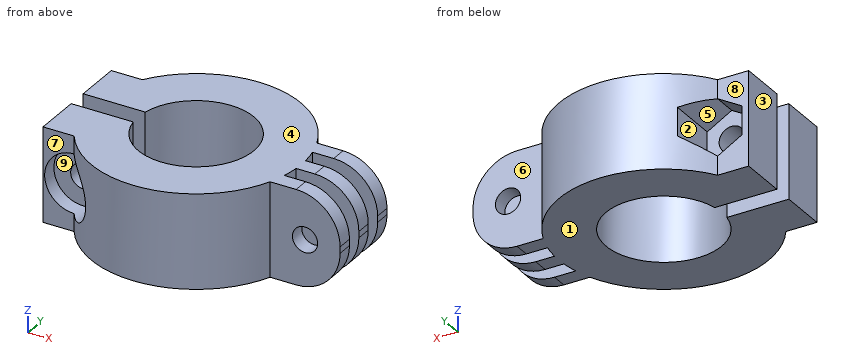
```python
from build123d import *

# Parameters (mm, degrees)
BODY_DEPTH                    = 19.05
SKETCH4_R                     = 5.9436
F_10_HEAD_CLEARANCE_DEPTH     = 49.85841003
F_10_NUT_CLEARANCE_DEPTH      = 51.814361521
F_10_NUT_CLEARANCE_DEPTH_BACK = 4.7625
FILLET2_R                     = 8.89
F_10_CLEARANCE_HOLE1_D        = 5.1054


with BuildPart() as part:
    # Sketch1 → Body (new body)
    with BuildSketch(Plane.XY):
        with BuildLine():
            ThreePointArc((-11.506493967, -2.02890428), (8.950462938, -7.510330831), (0, 11.684))
            ThreePointArc((0, 11.684), (-7.510330831, 8.950462938), (-11.506493967, 2.02890428))
            Line((-11.506493967, 2.02890428), (-24.064785284, 2.02890428))
            Line((-24.064785284, 2.02890428), (-24.064785284, 11.55390428))
            Line((-24.064785284, 11.55390428), (-17.785639626, 11.55390428))
            ThreePointArc((-17.785639626, 11.55390428), (21.209, 0), (-17.785639626, -11.55390428))
            Line((-17.785639626, -11.55390428), (-24.064785284, -11.55390428))
            Line((-24.064785284, -11.55390428), (-24.064785284, -2.02890428))
            Line((-24.064785284, -2.02890428), (-11.506493967, -2.02890428))
        make_face()
        with BuildLine():
            ThreePointArc((20.667372227, -4.7625), (20.229911928, -6.369642406), (19.667683513, -7.9375))
            Line((19.667683513, -7.9375), (33.849504125, -7.9375))
            Line((33.849504125, -7.9375), (33.849504125, -4.7625))
            Line((33.849504125, -4.7625), (20.667372227, -4.7625))
        make_face()
        with BuildLine():
            Line((33.849504125, 1.5875), (21.149504125, 1.5875))
            ThreePointArc((21.149504125, 1.5875), (21.209, 0), (21.149504125, -1.5875))
            Line((21.149504125, -1.5875), (33.849504125, -1.5875))
            Line((33.849504125, -1.5875), (33.849504125, 1.5875))
        make_face()
        with BuildLine():
            Line((33.849504125, 7.9375), (19.667683513, 7.9375))
            ThreePointArc((19.667683513, 7.9375), (20.229911928, 6.369642406), (20.667372227, 4.7625))
            Line((20.667372227, 4.7625), (33.849504125, 4.7625))
            Line((33.849504125, 4.7625), (33.849504125, 7.9375))
        make_face()
    extrude(amount=BODY_DEPTH)

    # Sketch3 → CBORE for #10 Binding Head Machine Screw1 (revolve, cut)
    with BuildSketch(Plane(origin=(-17.785639626, -11.55390428, 9.525), x_dir=(0, 0, -1), z_dir=(1, 0, 0))):
        Polygon((0, 0), (0, 32.76290428), (2.5527, 32.76290428), (2.5527, 3.1242), (5.9436, 3.1242), (5.9436, 0), align=None)
    revolve(axis=Axis((-17.785639626, -17.90390428, 9.525), (0, 1, 0)), mode=Mode.SUBTRACT)

    # Sketch4 → #10 Head clearance (cut, through all)
    with BuildSketch(Plane.XZ.offset(8.42970428)):
        with Locations(Location((-17.785639626, 9.525, 0), (0, 0, 270))):
            Circle(SKETCH4_R)
    extrude(amount=F_10_HEAD_CLEARANCE_DEPTH, mode=Mode.SUBTRACT)

    # Sketch5 → #10 nut clearance (cut, two sides: drawn at the far end of the back side and taken through both)
    with BuildSketch(Plane(origin=(0, 11.55390428, 0), x_dir=(1, 0, 0), z_dir=(0, 1, 0)).offset(-F_10_NUT_CLEARANCE_DEPTH_BACK)):
        with BuildLine():
            Line((-17.785639626, -3.805768233), (-22.738639626, -6.665384117))
            Line((-22.738639626, -6.665384117), (-22.738639626, -12.384615883))
            Line((-22.738639626, -12.384615883), (-17.785639626, -15.244231767))
            Line((-17.785639626, -15.244231767), (-17.785639626, -12.0777))
            ThreePointArc((-17.785639626, -12.0777), (-20.338339626, -9.525), (-17.785639626, -6.9723))
            Line((-17.785639626, -6.9723), (-17.785639626, -3.805768233))
        make_face()
        with BuildLine():
            Line((-12.832639626, -6.665384117), (-17.785639626, -3.805768233))
            Line((-17.785639626, -3.805768233), (-17.785639626, -6.9723))
            ThreePointArc((-17.785639626, -6.9723), (-20.338339626, -9.525), (-17.785639626, -12.0777))
            Line((-17.785639626, -12.0777), (-17.785639626, -15.244231767))
            Line((-17.785639626, -15.244231767), (-12.832639626, -12.384615883))
            Line((-12.832639626, -12.384615883), (-12.832639626, -6.665384117))
        make_face()
    extrude(amount=F_10_NUT_CLEARANCE_DEPTH + F_10_NUT_CLEARANCE_DEPTH_BACK, mode=Mode.SUBTRACT)

    # Fillet2
    fillet2_edges = [part.edges().sort_by_distance(p)[0] for p in [
        (33.849504125, 6.35, 0),
        (33.849504125, 0, 0),
        (33.849504125, -6.35, 0),
        (33.849504125, -6.35, 19.05),
        (33.849504125, 0, 19.05),
        (33.849504125, 6.35, 19.05),
    ]]
    fillet(fillet2_edges, radius=FILLET2_R)

    # #10 Clearance Hole1 (through all)
    with Locations(Plane(origin=(0, -7.9375, 0), x_dir=(-1, 0, 0), z_dir=(0, -1, 0))):
        with Locations((-26.758593819, -9.525)):
            Hole(F_10_CLEARANCE_HOLE1_D / 2)


solid = part.part
```
The model under review builds one solid part; all positions refer to its coordinate system, in mm. Face numbers are marked on the shaded views. A direction names the side the tool comes from. Give positions to 0.01 mm unless a question says otherwise; leave off trailing zeros. Write each loop counter-clockwise with the first axis right and the second up, starting at its lowest first coordinate (ties: lowest second). Pieces come first, ordered by that corner, then holes. Notation, with made-up numbers: M -40,32 L -18,32 A25 ccw -18,46 Z; hole C 22,75.5 d4. An arc over 180 degrees is marked long. Write item = value, one per line. Start each with the question number.
Q1. Mouldability with a two-part tool opening along Z and no side actions: class the marked faces 1, 2, 3 and 4 as released by +Z, released by -Z, zero draft, split by the parting line, or undercut.
Q2. Clearance check with flat-ended pins moving along their axes: pin 1 (4 mm diameter, centred on x = -17, z = 7, fed in from -Y); pin 2 (10 mm diameter, centred on x = -18.5, z = 13.5, fed in from +Y); pin 3 (4 mm diameter, centred on x = 26.76, z = 9.52, fed in from +Y); pin 4 (4 mm diameter, centred on y = -13, z = 6.5, fed in from +X). State where each tip first meets the part, or that it passes through.
Q3. Machinability: for the marked faces 5, 6, 7, 8 and 9, which of the approach directions +Z, -Z, +X, -X, +Y, -Y give a long, thin tool a straight path to every point of the face, cutting with its end or side? Answer none if there is none.
Q4. For line 1 (Y direction, x = 29.5, z = 13.25); line 2 (Y direction, x = -21.5, z = 6); line 3 (Y direction, x = 0, z = 11), list the stretches that pass through material, from the lowest coordinate up.
Q5. We need section C-C (x = 30.5). State the section outline as (y, z) points, plus the area to 3 significant figures.
Q6. We need section D-D (z = 5). State the section outline as (x, y) points, plus the area to 3 significant figures.
Q7. We need section B-B (y = 3). State the section outline as (x, z) points (3 decimals).
Q8. We need section A-A (x = 0). State the section outline as (y, z) points, plus the area to 3 significant figures.
Result set:
q1.face_1 = released by -Z
q1.face_2 = undercut
q1.face_3 = zero draft
q1.face_4 = released by +Z
q2.pin_1 = -8.43
q2.pin_2 = 16.36
q2.pin_3 = through
q2.pin_4 = 18.13
q3.face_5 = +Y
q3.face_6 = +Z, -Z, +X, +Y
q3.face_7 = +Z, -Z, -X, -Y
q3.face_8 = +Z, -Z, -X, +Y
q3.face_9 = -Y
q4.line_1 = -7.94 to -4.76, -1.59 to 1.59, 4.76 to 7.94
q4.line_2 = -8.43 to -2.03, 2.03 to 6.79
q4.line_3 = -21.21 to -11.68, 11.68 to 21.21
q5.outline = M -7.94,1.94 L -4.76,1.94 L -4.76,17.11 L -7.94,17.11 Z; M -1.59,1.94 L 1.59,1.94 L 1.59,17.11 L -1.59,17.11 Z; M 4.76,1.94 L 7.94,1.94 L 7.94,17.11 L 4.76,17.11 Z
q5.area = 145 mm2
q6.outline = M -24.06,-11.55 L -21.64,-11.55 L -21.64,-8.43 L -13.93,-8.43 L -13.93,-15.99 A21.21 ccw 19.67,-7.94 L 32.95,-7.94 L 32.95,-4.76 L 20.67,-4.76 A21.21 ccw 21.15,-1.59 L 32.95,-1.59 L 32.95,1.59 L 21.15,1.59 A21.21 ccw 20.67,4.76 L 32.95,4.76 L 32.95,7.94 L 19.67,7.94 A21.21 ccw -15.72,14.24 L -15.72,6.79 L -19.85,6.79 L -19.85,11.55 L -24.06,11.55 L -24.06,2.03 L -11.51,2.03 A11.68 cw long -11.51,-2.03 L -24.06,-2.03 Z
q6.area = 1,090 mm2
q7.outline = M -24.065,0 L -11.292,0 L -11.292,19.05 L -24.065,19.05 Z; M 11.292,0 L 20.996,0 L 20.996,19.05 L 11.292,19.05 Z; hole C -17.786,9.525 d5.105
q8.outline = M -21.21,0 L -11.68,0 L -11.68,19.05 L -21.21,19.05 Z; M 11.68,0 L 21.21,0 L 21.21,19.05 L 11.68,19.05 Z
q8.area = 363 mm2
